Geometry check sheet. Reference: the model listing, model coordinates, mm. Face numbers are marked on the shaded views. A direction names the side the tool comes from. Round coordinates to 2 decimals unless told otherwise and drop trailing zeros. Write each loop counter-clockwise with the first axis right and the second up, starting at its lowest first coordinate (ties: lowest second). Pieces come first, ordered by that corner, then holes.
Autodesk Inventor part; units mm, degrees
ref_plane "YZ Plane" through (0, 0, 0) normal (1, 0, 0) x (0, 1, 0)
ref_plane "XZ Plane" through (0, 0, 0) normal (0, 1, 0) x (-1, 0, 0)
ref_plane "XY Plane" through (0, 0, 0) normal (0, 0, 1) x (1, 0, 0)
sketch "Sketch1" plane through (0, 0, 0) normal (0, 0, 1) x (1, 0, 0)
  line L0 (-55, -30) -> (55, -30)
  line L1 (55, -30) -> (55, 30)
  line L2 (55, 30) -> (-55, 30)
  line L3 (-55, 30) -> (-55, -30)
  line L4 (-55, -30) -> (55, 30) construction
  line L5 (55, -30) -> (-55, 30) construction
  line L6 (0, -42) -> (0, 42)
  point P0 (0, 0)
  dimension "d1" = 110
  dimension "d2" = 60
  dimension "d60" = 0
extrude "Plate1" add sketch "Sketch1" along normal blind 3
sketch "Sketch2" plane through (0, 0, 3) normal (0, 0, 1) x (1, 0, 0)
  line L0 (26, -24) -> (50, -24)
  line L1 (50, -24) -> (50, -6)
  line L2 (50, -6) -> (26, -6)
  line L3 (26, -6) -> (26, -24)
  line L4 (26, -24) -> (50, -6) construction
  line L5 (50, -24) -> (26, -6) construction
  circle A0 centre (50, -6) radius 2.25
  circle A1 centre (50, -24) radius 2.25
  circle A2 centre (26, -24) radius 2.25
  circle A3 centre (26, -6) radius 2.25
  line L6 (55, 30) -> (55, -30)
  line L7 (55, -30) -> (-55, -30)
  point P0 (0, 0)
  point P1 (0, 0)
  point P2 (38, -15)
  dimension "d4" = 24
  dimension "d5" = 18
  dimension "d8" = 4.5
  dimension "d9" = 4.5
  dimension "d10" = 4.5
  dimension "d11" = 4.5
  dimension "d12" = 5
  dimension "d13" = 15
extrude "Cut1" cut sketch "Sketch2" against normal blind 3 contours L3 A2 L0 | L0 A2 L3 | A1 L1 L0 | L0 L1 A1 | A3 L2 L3 | L3 L2 A3 | A0 L2 L1 | L1 L2 A0
pattern_linear "Rectangular Pattern1" count 2 spacing 30 along (0, 1, 0) of "Cut1"
mirror "Mirror1" about plane through (0, 0, 0) normal (1, 0, 0) of "Cut1", "Rectangular Pattern1"
sketch "Sketch3" plane through (0, 0, 3) normal (0, 0, 1) x (1, 0, 0)
  line L0 (-12, -9) -> (12, -9)
  line L1 (12, -9) -> (12, 9)
  line L2 (12, 9) -> (-12, 9)
  line L3 (-12, 9) -> (-12, -9)
  line L4 (-12, -9) -> (12, 9) construction
  line L5 (12, -9) -> (-12, 9) construction
  circle A0 centre (-12, 9) radius 2.25
  circle A1 centre (12, 9) radius 2.25
  circle A2 centre (12, -9) radius 2.25
  circle A3 centre (-12, -9) radius 2.25
  line L6 (-77, 0) -> (77, 0)
  line L7 (0, -42) -> (0, 42)
  point P0 (0, 0)
  dimension "d20" = 24
  dimension "d21" = 18
  dimension "d22" = 4.5
  dimension "d23" = 4.5
  dimension "d24" = 4.5
  dimension "d25" = 4.5
  dimension "d26" = 12
  dimension "d27" = 9
extrude "Cut2" cut sketch "Sketch3" against normal blind 3 contours L3 A3 L0 | L0 A3 L3 | A2 L1 L0 | L0 L1 A2 | A0 L2 L3 | L3 L2 A0 | A1 L2 L1 | L1 L2 A1
sketch "Sketch4" plane through (0, 0, 3) normal (0, 0, 1) x (1, 0, 0)
  line L0 (-55, 30) -> (55, 30)
  line L1 (-22.5, 30) -> (22.5, 30)
  line L2 (22.5, 30) -> (22.5, 33)
  line L3 (22.5, 33) -> (-22.5, 33)
  line L4 (-22.5, 33) -> (-22.5, 30)
  point P0 (0, 0)
  point P1 (-50, 30)
  point P2 (50, 30)
  dimension "d30" = 45
  dimension "d31" = 3
  dimension "d32" = 22.5
sheet face with bend "Face2" sketch "Sketch4" thickness 3 toward (0, 0, -1) bend radius 3
bend "Bend1"
sketch "Sketch5" plane through (-22.5, 33, 3) normal (0, 1, 0) x (-1, 0, 0)
  line L0 (-45, 0) -> (0, 0)
  line L1 (0, 0) -> (0, 52)
  line L2 (0, 52) -> (-45, 52)
  line L3 (-45, 52) -> (-45, 0)
edge flange "Flange1" height 55 angle 90 thickness 3 bend radius 3 thickness toward (0, 1, 0) relief tear relief width 3 relief depth 1.5 edges at (0, 33, 3) wall of the first edge with corners at (22.5, 33, 3) (-22.5, 33, 3) (-22.5, 33, 55) (22.5, 33, 55)
bend "Bend2"
corner "Corner1"
sketch "Sketch6" plane through (-22.5, 36, 55) normal (0, 1, 0) x (1, 0, 0)
  circle A0 centre (22.5, 22) radius 9
  line L0 (0, 55) -> (45, 55)
  circle A1 centre (37.5, 22) radius 2.25
  circle A2 centre (8.5, 22) radius 2.25
  line L1 (45, 49) -> (45, 0)
  line L2 (45, 55) -> (0, 55)
  point P0 (22.5, 55)
  point P1 (-25, 55)
  dimension "d48" = 18
  dimension "d49" = 33
  dimension "d50" = 4.5
  dimension "d51" = 4.5
  dimension "d52" = 29
  dimension "d53" = 22.5
  dimension "d54" = 15
  dimension "d55" = 33
  dimension "d56" = 33
extrude "Cut3" cut sketch "Sketch6" against normal blind 3
fillet "Fillet2" radius 10 2 edges at (22.5, 34.5, 55) (-22.5, 34.5, 55)
fillet "Fillet4" radius 3 4 edges at (55, 30, 1.5) (55, -30, 1.5) (-55, -30, 1.5) (-55, 30, 1.5)
equation "\"d14\" = Thickness"
equation "\"d28\" = Thickness"
equation "\"d57\" = Thickness"
equation "\"d3\" = Thickness"
equation "\"d33\" = BendRadius"
equation "\"d34\" = BendReliefWidth"
equation "\"d36\" = MinimumRemnant"
equation "\"d35\" = BendReliefDepth"
equation "\"d37\" = TransitionRadius"
equation "\"d38\" = BendReliefWidth"
equation "\"d39\" = BendReliefDepth"
equation "\"d40\" = MinimumRemnant"
equation "\"d41\" = TransitionRadius"
equation "\"d44\" = BendRadius"
equation "\"d45\" = CornerReliefSize"
equation "\"d46\" = GapSize"
equation "\"d47\" = JacobiRadiusSize"
equation "\"BendRadius\" = Thickness"
equation "\"BendReliefWidth\" = Thickness"
equation "\"BendReliefDepth\" = 0.5 * Thickness"
equation "\"CornerReliefSize\" = 4 * Thickness"
equation "\"MinimumRemnant\" = 2 * Thickness"
equation "\"TransitionRadius\" = BendRadius"
equation "\"JacobiRadiusSize\" = BendRadius"
equation "\"GapSize\" = Thickness"
properties part number "De truc Z chan sat"
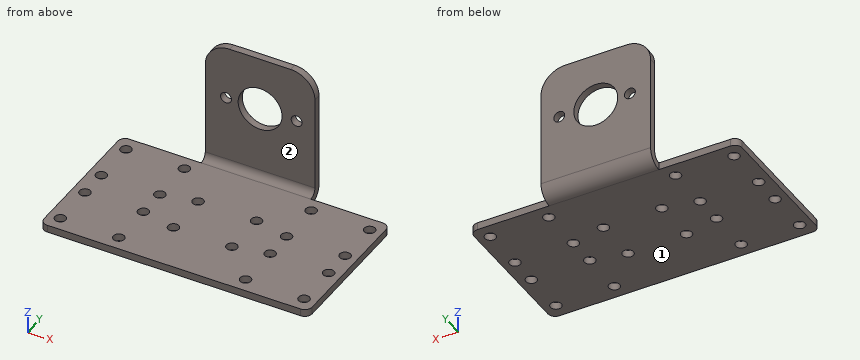
1. Scan lines: line 1 along X through (y, z) = (6, 2.45); line 2 along X through (y, z) = (35, 33); line 3 along Y through (x, z) = (50, 1). Record each from-to range of solid material in increasing order.
2. Section check B-B (x = 0). Record the cut outline in (y, z).
3. Depth check by flat-ended pin: pin 1 Ø4 at (x, y) = (-12, 9) entering from +Z; pin 2 Ø1.5 at (x, y) = (43, -6) entering from -Z; pin 3 Ø1.5 at (x, z) = (35.5, 1) entering from +Y; pin 4 Ø1 at (x, y) = (-26, -19.5) entering from +Z. Enter the tip coordinate at first touch or a pass-through.
4. Section check C-C (y = 0). Record the cut outline in (x, z), plus the area to 3 significant figures.
5. Access from +Z, -Z, +X, -X, +Y, -Y to the whole of each face (thin tool, end or side, straight path). Record for the marked faces 1 and 2.
6. Section check A-A (z = 33). Record the cut outline in (x, y).
7. Section check D-D (x = 21). Record the cut outline in (y, z).
Results below:
1. line 1: x = -55 to -52.25, -47.75 to -28.25, -23.75 to 23.75, 28.25 to 47.75, 52.25 to 55
1. line 2: x = -22.5 to -16.25, -11.75 to -9, 9 to 12.75, 17.25 to 22.5
1. line 3: y = -30 to -26.25, -21.75 to -8.25, -3.75 to 3.75, 8.25 to 21.75, 26.25 to 30
2. outline: (-30, 0) - (30, 0) arc R6 ccw to (36, 6) - (36, 24) - (33, 24) - (33, 6) arc R3 cw to (30, 3) - (-30, 3) - close; (33, 42) - (36, 42) - (36, 55) - (33, 55) - close
3. pin 1: passes through
3. pin 2: stops at z = 0
3. pin 3: stops at y = 30
3. pin 4: stops at z = 3
4. outline: (-55, 0) - (55, 0) - (55, 3) - (-55, 3) - close
4. area: 330 mm2
5. face 1: -Z, +X, -X, +Y, -Y
5. face 2: +Z, +X, -X, -Y
6. outline: (-22.5, 33) - (-16.25, 33) - (-16.25, 36) - (-22.5, 36) - close; (-11.75, 33) - (-9, 33) - (-9, 36) - (-11.75, 36) - close; (9, 33) - (12.75, 33) - (12.75, 36) - (9, 36) - close; (17.25, 33) - (22.5, 33) - (22.5, 36) - (17.25, 36) - close
7. outline: (-30, 0) - (30, 0) arc R6 ccw to (36, 6) - (36, 50.27) - (33, 50.27) - (33, 6) arc R3 cw to (30, 3) - (-30, 3) - close
